from build123d import *

# Parameters (mm, degrees)
SKETCH1_W                  = 130
SKETCH1_H                  = 100
BOSS_EXTRUDE1_DEPTH        = 20
SKETCH2_W                  = 130
SKETCH2_H                  = 20
BOSS_EXTRUDE2_DEPTH        = 70
FILLET1_R                  = 20
SKETCH3_W                  = 60
SKETCH3_H                  = 70
BOSS_EXTRUDE3_DEPTH        = 50
CUT_EXTRUDE1_DEPTH         = 132.244047484
CHAMFER1_SIZE              = 30
F_10_0_10_DIAMETER_HOLE1_D = 10
F_15_0_15_DIAMETER_HOLE1_D = 15
FILLET2_R                  = 5


with BuildPart() as part:
    # Sketch1 → Boss-Extrude1 (new body)
    with BuildSketch(Plane(origin=(0, 0, 0), x_dir=(1, 0, 0), z_dir=(0, 1, 0))):
        Rectangle(SKETCH1_W, SKETCH1_H)
    extrude(amount=BOSS_EXTRUDE1_DEPTH)

    # Sketch2 → Boss-Extrude2 (add)
    with BuildSketch(Plane(origin=(0, 20, 0), x_dir=(1, 0, 0), z_dir=(0, 1, 0))):
        with Locations((0, 40)):
            Rectangle(SKETCH2_W, SKETCH2_H)
    extrude(amount=BOSS_EXTRUDE2_DEPTH)

    # Fillet1
    fillet1_edges = [part.edges().sort_by_distance(p)[0] for p in [
        (-65, 10, 50),
        (-65, 90, -40),
    ]]
    fillet(fillet1_edges, radius=FILLET1_R)

    # Sketch3 → Boss-Extrude3 (add)
    with BuildSketch(Plane.XY.offset(-30)):
        with Locations((35, 55)):
            Rectangle(SKETCH3_W, SKETCH3_H)
    extrude(amount=BOSS_EXTRUDE3_DEPTH)

    # Sketch4 → Cut-Extrude1 (cut, through all)
    with BuildSketch(Plane.XY.offset(20)):
        with BuildLine():
            Line((40, 90), (40, 55))
            ThreePointArc((40, 55), (47.32233047, 37.32233047), (65, 30))
            Line((65, 30), (65, 90))
            Line((65, 90), (40, 90))
        make_face()
    extrude(amount=-CUT_EXTRUDE1_DEPTH, mode=Mode.SUBTRACT)

    # Chamfer1
    chamfer1_edges = [part.edges().sort_by_distance(p)[0] for p in [
        (22.5, 90, 20),
    ]]
    chamfer(chamfer1_edges, length=CHAMFER1_SIZE)

    # Ø10.0 (10) Diameter Hole1 (through all)
    with Locations(Plane.ZY.offset(-5)):
        with Locations((-10, 65)):
            Hole(F_10_0_10_DIAMETER_HOLE1_D / 2)

    # Ø15.0 (15) Diameter Hole1 (through all)
    with Locations(Plane(origin=(0, 20, 0), x_dir=(1, 0, 0), z_dir=(0, 1, 0))):
        with Locations((-45, -30)):
            Hole(F_15_0_15_DIAMETER_HOLE1_D / 2)

    # Fillet2
    fillet2_edges = [part.edges().sort_by_distance(p)[0] for p in [
        (-65, 20, 0),
        (10, 20, 50),
        (-65, 35, -50),
        (-2.5, 90, -50),
        (-20, 90, -30),
        (-65, 45, -30),
        (-59.142135624, 20, 44.142135624),
        (-59.142135624, 84.142135624, -50),
        (-59.142135624, 84.142135624, -30),
        (-30, 20, -30),
    ]]
    fillet(fillet2_edges, radius=FILLET2_R)


solid = part.part
Read the model definition and answer for the solid it produces. Units are mm, in the model's axes. A direction names the side the tool comes from. Give positions to 0.01 mm unless a question says otherwise; leave off trailing zeros. Write each loop counter-clockwise with the first axis right and the second up, starting at its lowest first coordinate (ties: lowest second). Pieces come first, ordered by that corner, then holes. Notation, with made-up numbers: M -28.5,77 L 24.5,77 A17 ccw 24.5,107 Z; hole C 85,30.5 d7. An arc over 180 degrees is marked long. One line per item, written item: value. Start each with the question number.
(1) Find the intervals of material crossed by line 1 (Z direction, x = -45, y = 7.5); line 2 (Y direction, x = 25, z = -10); line 3 (Z direction, x = 24, y = 30), in increasing order.
(2) Determine the mould class of faces 1 (the cylindrical face through (-27, 22, -29)), 2 (the cylindrical face through (23, 69, -13)), 3 (the flat face through (5, 47, -8)) for opening direction Y: pulls with the +Y half, pulls with the -Y half, needs draft (parallel to the pull), parting line crosses it, or undercut.
(3) Flat-ended cylindrical pins translate along their axes: pin 1 Ø1.5 at (x, y) = (23, 75) entering from +Z; pin 2 Ø12 at (x, y) = (21, 35.5) entering from +Z; pin 3 Ø18 at (x, y) = (-33.5, 46.5) entering from +Z; pin 4 Ø13.5 at (x, z) = (-45, 30) entering from +Y. Find the tip coordinate at first contact, or state that the pin passes through.
(4) Find section B-B (x = 22). Determine the outline of the cut face in (y, z).
(5) Find section C-C (z = 17). Determine the outline of the cut face in (x, y), plus the area to 3 significant figures.
(6) Find section A-A (y = 65). Determine the outline of the cut face in (x, z), plus the area to 3 significant figures.
(7) A tool of negligible diameter and unlimited length cuts with its end or side. For faces 4 (the flat face through (-12, 42, -50)), 5 (the flat face through (-28, 55, -30)), from which of +Z, -Z, +X, -X, +Y, -Y can it reach the whole face along a straight path? Write none if from no direction.
(8) Find section D-D (y = 7.5). Determine the outline of the cut face in (x, z), plus the area to 3 significant figures.
Results below:
1. line 1: z = -50 to 22.5, 37.5 to 50
1. line 2: y = 0 to 60, 70 to 90
1. line 3: z = -50 to 20
2. face 1: pulls with the +Y half
2. face 2: undercut
2. face 3: needs draft
3. pin 1: stops at z = 5.75
3. pin 2: stops at z = 20
3. pin 3: stops at z = -30
3. pin 4: passes through
4. outline: M 0,-50 L 85,-50 A5 ccw 90,-45 L 90,-10 L 60,20 L 20,20 L 20,45 A5 ccw 15,50 L 0,50 Z; hole C 65,-10 d10
5. outline: M -65,0 L 65,0 L 65,30 A25 cw 40,55 L 40,63 L 5,63 L 5,20 L -60,20 A5 ccw -65,15 Z
5. area: 4,480 mm^2
6. outline: M -65,-45 A5 ccw -60,-50 L 40,-50 L 40,-15 L 5,-15 L 5,-30 L -60,-30 A5 ccw -65,-35 Z; M 5,-5 L 40,-5 L 40,15 L 5,15 Z
6. area: 3,310 mm^2
7. face 4: -Z, +X, -X, +Y, -Y
7. face 5: +Z, -X, +Y
8. outline: M -65,-45 A5 ccw -60,-50 L 65,-50 L 65,50 L -45,50 A20 ccw -65,30 Z; hole C -45,30 d15
8. area: 12,700 mm^2
